Part model, mm, in its own coordinate system. Face numbers are marked on the shaded views. Coordinates: 2 decimals unless noted, no trailing zeros. Loops run counter-clockwise (first coordinate to the right, second up) from the corner with the lowest first, then second, coordinate; pieces in that order, holes last. Notation, with made-up numbers: (-33, 51.25) - (-15, 51.25) arc R20 cw to (-15, 83.25) - close; hole circle Ø8 at (84.5, -13). An arc over 180 degrees is marked (long way). Use a Markdown table: item, result. Add a question column.
1) Band-saw the part on A-A (z = 3). Give the cut face in (x, y), plus the area to 3 significant figures.
2) Drop flat-ended pins along their axis: P1, Ø5, axis at x = -0.41, z = 1.55, coming from the +Y side; P2, Ø1.5, axis at x = 1, y = -1, coming from the -Z side; P3, Ø2.5, axis at x = -0.41, z = -3.46, coming from the -Y side. Give the stop position or say it passes through.
3) Probe probe 1 along Z at (x, y) = (0.25, 1.45); probe 2 along X at (y, z) = (0.95, -4.5); probe 3 along X at (y, z) = (0.05, 1). List the from-to ranges inside material, lowest first. Write a range as [from, to].
4) Band-saw the part on D-D (x = -4.5). Give the cut face in (y, z), plus the area to 3 significant figures.
5) Pull direction X, two halves, no side cores. Call the marked faces 1, 2, 3 and 4: +X half, -X half, draft (parallel to the pull), parting line (faces both ways), or undercut.
6) Band-saw the part on B-B (x = 0.25). Give the number of separate pieces and of enclosed holes in the cut face, plus the area to 3 significant figures.
7) Band-saw the part on C-C (y = 1.45). Give the cut face in (x, z) (1 decimal).
from build123d import *

# Parameters (mm, degrees)
F0_R     = 1.1811
F0_R_2   = 1.5875
F1_DEPTH = 1.5875
F2_SIZE2 = 0.254
F2_SIZE  = 0.254
F3_SIZE  = 0.508


with BuildPart() as f1:
    # F0 (on Front) → F1 (new body, symmetric)
    with BuildSketch(Plane.XZ):
        with BuildLine():
            Line((5.750813, 4.094138), (-6.573008, 4.094138))
            ThreePointArc((-6.573008, 4.094138), (-4.49461, -3.713278), (3.584436, -3.780322))
            Line((3.584436, -3.780322), (5.750813, 4.094138))
        make_face()
        with Locations((-0.411098, -3.459583)):
            Circle(F0_R, mode=Mode.SUBTRACT)
        with Locations((-0.411098, 1.554138)):
            Circle(F0_R_2, mode=Mode.SUBTRACT)
    extrude(amount=F1_DEPTH, both=True)

    # F2
    f2_edges = [f1.edges().sort_by_distance(p)[0] for p in [
        (-1.592198, -1.5875, -3.459583),
    ]]
    chamfer(f2_edges, length=F2_SIZE, length2=F2_SIZE2)

    # F3
    f3_edges = [f1.edges().sort_by_distance(p)[0] for p in [
        (5.750813, 0, 4.094138),
    ]]
    chamfer(f3_edges, length=F3_SIZE)


solid = f1.part
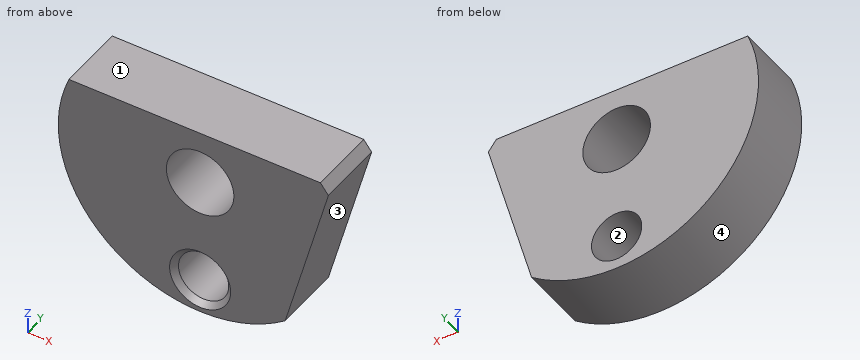
Answer block:
| question | item | result |
|---|---|---|
| 1 | outline | (-6.92, -1.59) - (-1.07, -1.59) - (-1.07, 1.59) - (-6.92, 1.59) - close; (0.24, -1.59) - (5.45, -1.59) - (5.45, 1.59) - (0.24, 1.59) - close |
| 1 | area | 35.1 mm2 |
| 2 | P1 | y = 1.59 |
| 2 | P2 | z = -5.08 |
| 2 | P3 | y = -1.4 |
| 3 | probe 1 | [-5.08, -4.44], [-2.48, 0.11], [3, 4.09] |
| 3 | probe 2 | [-3.2, -0.97], [0.15, 2.38] |
| 3 | probe 3 | [-7.05, -1.9], [1.08, 4.9] |
| 4 | outline | (-1.59, -3.71) - (1.59, -3.71) - (1.59, 4.09) - (-1.59, 4.09) - close |
| 4 | area | 24.8 mm2 |
| 5 | face 1 | draft |
| 5 | face 2 | undercut |
| 5 | face 3 | +X half |
| 5 | face 4 | parting line |
| 6 | separate pieces | 3 |
| 6 | enclosed holes | 0 |
| 6 | area | 13.7 mm2 |
| 7 | outline | (-6.6, 4.1) arc R6.7 ccw to (3.6, -3.8) - (5.6, 3.6) - (5.2, 4.1) - close; hole circle Ø3.2 at (-0.4, 1.6); hole circle Ø2.4 at (-0.4, -3.5) |
